Autodesk Inventor part; units mm, degrees
ref_plane "YZ Plane" through (0, 0, 0) normal (1, 0, 0) x (0, 1, 0)
ref_plane "XZ Plane" through (0, 0, 0) normal (0, 1, 0) x (-1, 0, 0)
ref_plane "XY Plane" through (0, 0, 0) normal (0, 0, 1) x (1, 0, 0)
sketch "스케치1" plane through (0, 0, 0) normal (1, 0, 0) x (0, 1, 0)
  circle A0 centre (0, 0) radius 37
  dimension "d0" = 74
extrude "돌출1" add sketch "스케치1" along normal blind 24
sketch "스케치2" plane through (24, 0, 0) normal (1, 0, 0) x (0, 0, -1)
  circle A0 centre (0, 0) radius 5
  dimension "d3" = 10
extrude "돌출2" cut sketch "스케치2" against normal blind 24
sketch "스케치3" plane through (24, 0, 0) normal (1, 0, 0) x (0, 0, -1)
  circle A0 centre (0, 0) radius 5
  circle A1 centre (0, 0) radius 16
extrude "돌출4" cut sketch "스케치3" against normal blind 19
sketch "스케치4" plane through (5, 0, 0) normal (1, 0, 0) x (0, 0, -1)
  circle A0 centre (-10, 0) radius 1.75
  circle A1 centre (0, 10) radius 1.75
  circle A2 centre (10, 0) radius 1.75
  circle A3 centre (0, -10) radius 1.75
  point P0 (0, 0)
  dimension "d21" = 3.5
  dimension "d22" = 3.5
  dimension "d23" = 3.5
  dimension "d24" = 3.5
extrude "돌출5" cut sketch "스케치4" against normal blind 19
sketch "스케치5" plane through (24, 0, 0) normal (1, 0, 0) x (0, 0, -1)
  circle A0 centre (0, 0) radius 19
  circle A1 centre (0, 0) radius 32
  line L0 (0, 0) -> (-22.6274, 22.6274)
  line L1 (0, 0) -> (32, 0) construction
  line L2 (-22.6274, 22.6274) -> (22.6274, -22.6274)
  line L3 (0, 0) -> (-22.6274, -22.6274)
  line L4 (0, 0) -> (32, 0) construction
  line L5 (-22.6274, -22.6274) -> (22.6274, 22.6274)
  line L6 (-18, 18) -> (-16.5858, 19.4142)
  line L7 (-16.5858, 19.4142) -> (-19.4142, 16.5858)
  line L8 (-16.5858, 19.4142) -> (-11.9462, 14.7746)
  line L9 (-21.169, 23.9974) -> (-16.5858, 19.4142)
  line L10 (-19.4142, 16.5858) -> (-23.9974, 21.169)
  line L11 (-14.7746, 11.9462) -> (-19.4142, 16.5858)
  line L12 (18, 18) -> (16.5858, 19.4142)
  line L13 (16.5858, 19.4142) -> (19.4142, 16.5858)
  line L14 (19.4142, 16.5858) -> (14.7746, 11.9462)
  line L15 (23.9974, 21.169) -> (19.4142, 16.5858)
  line L16 (16.5858, 19.4142) -> (21.169, 23.9974)
  line L17 (16.5858, 19.4142) -> (11.9462, 14.7746)
  line L18 (18, -18) -> (19.4142, -16.5858)
  line L19 (19.4142, -16.5858) -> (16.5858, -19.4142)
  line L20 (16.5858, -19.4142) -> (11.9462, -14.7746)
  line L21 (16.5858, -19.4142) -> (21.169, -23.9974)
  line L22 (19.4142, -16.5858) -> (14.7746, -11.9462)
  line L23 (19.4142, -16.5858) -> (23.9974, -21.169)
  line L24 (-18, -18) -> (-19.4142, -16.5858)
  line L25 (-19.4142, -16.5858) -> (-16.5858, -19.4142)
  line L26 (-16.5858, -19.4142) -> (-11.9462, -14.7746)
  line L27 (-16.5858, -19.4142) -> (-21.169, -23.9974)
  line L28 (-19.4142, -16.5858) -> (-14.7746, -11.9462)
  line L29 (-23.9974, -21.169) -> (-19.4142, -16.5858)
  dimension "d27" = 38
  dimension "d28" = 64
  dimension "d29" = 135
  dimension "d30" = 135
  dimension "d31" = 2
  dimension "d32" = 4
  dimension "d33" = 2
extrude "돌출6" cut sketch "스케치5" against normal blind 19 contours A0 L14 L15 A1 L23 L22 | A0 L8 L9 A1 L16 L17 | L20 L21 A1 L27 L26 A0 | A0 L28 L29 A1 L10 L11
sketch "스케치6" plane through (24, 0, 0) normal (1, 0, 0) x (0, 0, -1)
  circle A0 centre (0, 0) radius 35
  circle A1 centre (0, 0) radius 37
  dimension "d36" = 70
  dimension "d37" = 74
extrude "돌출7" cut sketch "스케치6" against normal blind 22
properties part number "바퀴" material "아세탈 수지, 검은색"
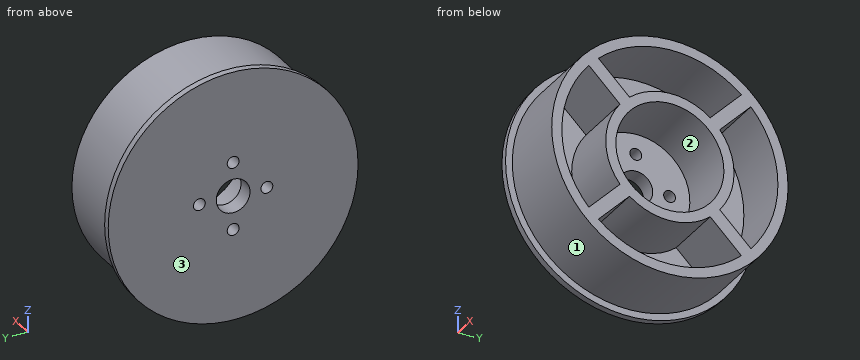
Geometry: final body of the model. Coordinates: model frame, mm. Face numbers are marked on the shaded views. Round coordinates to 2 decimals unless told otherwise and drop trailing zeros. Order: outer loops, then holes, each group sorted by start corner. A loop starts at its lowest first (then second) coordinate and runs counter-clockwise, first axis right, second up. Notation, with made-up numbers: (62.25, 3.5) -> (101.25, 3.5) arc R30 cw to (101.25, 36.5) -> close; hole circle Ø9 at (-25, 42). An arc over 180 degrees is marked (long way). Use CSV: the item, a comma, the result in double quotes. Start each with the question number.
1) Section B-B (y = 10). Return the cut outline in (x, z).
2) Section D-D (x = 14.75). Return the cut outline in (y, z), and give its area (3 significant figures).
3) Material intervals for line 1 along Y through (x, z) = (1.05, 0); line 2 along Y through (x, z) = (10, -0.5); line 3 along Z through (x, y) = (14.75, -20), sorted ascending. Write a range as from..to.
4) Section A-A (z = 0). State how many separate pieces and enclosed holes the cut face has, and give its area (3 significant figures).
5) First-contact query: pin 1 Ø3 at (y, z) = (10, 0) entering from -X; pin 2 Ø4 at (x, z) = (3, 12) entering from -Y; pin 3 Ø1 at (x, y) = (16, 23) entering from -Z; pin 4 Ø12 at (x, y) = (16, 13.5) entering from -Z. Flat tips, straight axial feed; report the tip coordinate or a pass-through.
6) Draft query along Z for the marked faces 1, 2 and 3. Return one class per face: +Z half, -Z half, draft (parallel to the pull), parting line (faces both ways), or undercut.
Returned:
1,outline,"(0, -35.62) -> (2, -35.62) -> (2, -33.54) -> (24, -33.54) -> (24, -30.4) -> (5, -30.4) -> (5, -16.16) -> (24, -16.16) -> (24, -12.49) -> (5, -12.49) -> (5, -1.75) -> (0, -1.75) -> close; (0, 1.75) -> (5, 1.75) -> (5, 12.49) -> (24, 12.49) -> (24, 16.16) -> (5, 16.16) -> (5, 30.4) -> (24, 30.4) -> (24, 33.54) -> (2, 33.54) -> (2, 35.62) -> (0, 35.62) -> close"
2,outline,"circle Ø70 at (0, 0); hole (-24, -21.17) -> (-14.77, -11.95) arc R19 cw to (-14.77, 11.95) -> (-24, 21.17) arc R32 ccw to start; hole (-21.17, -24) arc R32 ccw to (21.17, -24) -> (11.95, -14.77) arc R19 cw to (-11.95, -14.77) -> close; hole (-21.17, 24) -> (-11.95, 14.77) arc R19 cw to (11.95, 14.77) -> (21.17, 24) arc R32 ccw to start; hole circle Ø32 at (0, 0); hole (14.77, -11.95) -> (24, -21.17) arc R32 ccw to (24, 21.17) -> (14.77, 11.95) arc R19 cw to start"
2,area,"1,170 mm²"
3,line 1,"y = -37..-11.75, -8.25..-5, 5..8.25, 11.75..37"
3,line 2,"y = -35..-32, -18.99..-15.99, 15.99..18.99, 32..35"
3,line 3,"z = -28.72..-24.98, -22.83..-17.17, 17.17..22.83, 24.98..28.72"
4,separate pieces,"4"
4,enclosed holes,"0"
4,area,"501 mm²"
5,pin 1,"passes through"
5,pin 2,"stops at y = -35.55"
5,pin 3,"stops at z = -26.81"
5,pin 4,"stops at z = -34.19"
6,face 1,"parting line"
6,face 2,"undercut"
6,face 3,"draft"
